Build history of the part. All positions in model axes, mm. A direction names the side the tool comes from. Round coordinates to 2 decimals unless told otherwise and drop trailing zeros. Write each loop counter-clockwise with the first axis right and the second up, starting at its lowest first coordinate (ties: lowest second). Pieces come first, ordered by that corner, then holes. Notation, with made-up numbers: (-35, -32.75) -> (-14, -32.75) arc R17 ccw to (-14, -1.75) -> close; hole circle Ø1 at (79, 69). An arc over 180 degrees is marked (long way). One line per question, with ' | ' between items.
from build123d import *

# Parameters (mm, degrees)
SKETCH1_R           = 11
SKETCH1_R_2         = 1.25
SKETCH1_R_3         = 2.5
SKETCH1_R_4         = 2.1
BOSS_EXTRUDE1_DEPTH = 2.5
FILLET1_R           = 0.5
FILLET2_R           = 2


with BuildPart() as part:
    # Sketch1 → Boss-Extrude1 (new, symmetric)
    with BuildSketch(Plane.XY):
        with BuildLine():
            Line((-30, -46), (-22.5, -46))
            Line((-22.5, -46), (-22.5, -45.3))
            ThreePointArc((-22.5, -45.3), (-23.8, -44), (-22.5, -42.7))
            Line((-22.5, -42.7), (-20.5, -42.7))
            ThreePointArc((-20.5, -42.7), (-19.2, -44), (-20.5, -45.3))
            Line((-20.5, -45.3), (-20.5, -46))
            Line((-20.5, -46), (20.5, -46))
            Line((20.5, -46), (20.5, -45.3))
            ThreePointArc((20.5, -45.3), (19.2, -44), (20.5, -42.7))
            Line((20.5, -42.7), (22.5, -42.7))
            ThreePointArc((22.5, -42.7), (23.8, -44), (22.5, -45.3))
            Line((22.5, -45.3), (22.5, -46))
            Line((22.5, -46), (30, -46))
            Line((30, -46), (30, 49))
            ThreePointArc((30, 49), (0, 79), (-30, 49))
            Line((-30, 49), (-30, -46))
        make_face()
        with Locations((0, -4.6)):
            Circle(SKETCH1_R, mode=Mode.SUBTRACT)
        with Locations((15.5, 10.9)):
            Circle(SKETCH1_R_2, mode=Mode.SUBTRACT)
        with Locations((15.5, -20.1)):
            Circle(SKETCH1_R_2, mode=Mode.SUBTRACT)
        with Locations((-15.5, -20.1)):
            Circle(SKETCH1_R_2, mode=Mode.SUBTRACT)
        with Locations((-15.5, 10.9)):
            Circle(SKETCH1_R_2, mode=Mode.SUBTRACT)
        with Locations((0, 49)):
            Circle(SKETCH1_R, mode=Mode.SUBTRACT)
        with Locations((21.5, -34)):
            Circle(SKETCH1_R_3, mode=Mode.SUBTRACT)
        with Locations((-21.5, -34)):
            Circle(SKETCH1_R_3, mode=Mode.SUBTRACT)
        with Locations((0, 64)):
            Circle(SKETCH1_R_4, mode=Mode.SUBTRACT)
        with Locations((-15, 49)):
            Circle(SKETCH1_R_4, mode=Mode.SUBTRACT)
        with Locations((0, 34)):
            Circle(SKETCH1_R_4, mode=Mode.SUBTRACT)
        with Locations((15, 49)):
            Circle(SKETCH1_R_4, mode=Mode.SUBTRACT)
        with Locations((20, 19.25)):
            Circle(SKETCH1_R_4, mode=Mode.SUBTRACT)
        with BuildLine():
            Line((20.5, -26.5), (22.5, -26.5))
            ThreePointArc((22.5, -26.5), (24, -28), (22.5, -29.5))
            Line((22.5, -29.5), (20.5, -29.5))
            ThreePointArc((20.5, -29.5), (19, -28), (20.5, -26.5))
        make_face(mode=Mode.SUBTRACT)
        with BuildLine():
            Line((-20.5, -26.5), (-22.5, -26.5))
            ThreePointArc((-22.5, -26.5), (-24, -28), (-22.5, -29.5))
            Line((-22.5, -29.5), (-20.5, -29.5))
            ThreePointArc((-20.5, -29.5), (-19, -28), (-20.5, -26.5))
        make_face(mode=Mode.SUBTRACT)
        with BuildLine():
            Line((-8.51843153, 12.888546871), (-18.855050358, 16.650768448))
            ThreePointArc((-18.855050358, 16.650768448), (-20.349231552, 19.855050358), (-17.144949642, 21.349231552))
            Line((-17.144949642, 21.349231552), (-6.808330813, 17.587009975))
            ThreePointArc((-6.808330813, 17.587009975), (-5.314149619, 14.382728065), (-8.51843153, 12.888546871))
        make_face(mode=Mode.SUBTRACT)
    extrude(amount=BOSS_EXTRUDE1_DEPTH, both=True)

    # Fillet1
    # the kernel refuses this fillet: 0.5 mm, written as the material it takes off along each edge
    with BuildSketch(Plane(origin=(-22.5, -46, -3.75), x_dir=(0, 1, 0), z_dir=(0, 0, 1)), Plane(origin=(-20.5, -46, -3.75), x_dir=(1, 0, 0), z_dir=(0, 0, 1)), Plane(origin=(20.5, -46, -3.75), x_dir=(0, 1, 0), z_dir=(0, 0, 1)), Plane(origin=(22.5, -46, -3.75), x_dir=(1, 0, 0), z_dir=(0, 0, 1))) as fillet1_piece_1:
        with BuildLine():
            CenterArc((FILLET1_R, FILLET1_R), FILLET1_R, 180, 90)
            Line((0, FILLET1_R), (0, 0))
            Line((0, 0), (FILLET1_R, 0))
        make_face()
    extrude(amount=7.5, mode=Mode.SUBTRACT)
    with BuildSketch(Plane(origin=(-22.5, -45.3, -3.572904116), x_dir=(-0.990112458059838, 0.14027587246103826, 0), z_dir=(0, 0, 1))) as fillet1_piece_2:
        with BuildLine():
            CenterArc((0.434855205, 0.495056229), FILLET1_R, 188.063810107, 73.872379787)
            Line((-0.060201024, 0.424918293), (0, 0))
            ThreePointArc((0, 0), (0.182358634, 0.012853805), (0.364717268, 0))
        make_face()
    extrude(amount=7.145808233, mode=Mode.SUBTRACT)
    with BuildSketch(Plane(origin=(-20.5, -45.3, -3.572904116), x_dir=(0, -1, 0), z_dir=(0, 0, 1))) as fillet1_piece_3:
        with BuildLine():
            CenterArc((0.429161647, 0.5), FILLET1_R, 196.127620213, 73.872379787)
            ThreePointArc((-0.051161033, 0.361111111), (-0.012853805, 0.182358634), (0, 0))
            Line((0, 0), (0.429161647, 0))
        make_face()
    extrude(amount=7.145808233, mode=Mode.SUBTRACT)
    with BuildSketch(Plane(origin=(20.5, -45.3, 3.572904116), x_dir=(-0.9901124580598404, 0.14027587246102047, 0), z_dir=(0, 0, -1)), Plane(origin=(22.5, -45.3, -3.572904116), x_dir=(0.9901124580598378, 0.1402758724610396, 0), z_dir=(0, 0, 1))) as fillet1_piece_4:
        with BuildLine():
            CenterArc((0.434855205, -0.495056229), FILLET1_R, 98.063810107, 73.872379787)
            Line((-0.060201024, -0.424918293), (0, 0))
            ThreePointArc((0, 0), (0.182358634, -0.012853805), (0.364717268, 0))
        make_face()
    extrude(amount=7.145808233, mode=Mode.SUBTRACT)

    # Fillet2
    fillet2_edges = [part.edges().sort_by_distance(p)[0] for p in [
        (30, -46, 0),
        (-30, -46, 0),
    ]]
    fillet(fillet2_edges, radius=FILLET2_R)


solid = part.part
(1) Wall check: line 1 (Y direction, x = 0, z = -0.7); line 2 (Y direction, x = 16, z = 0.3); line 3 (Y direction, x = -15.5, z = -0.85). Give the ranges that are in metal, low to high. Write a range as from..to.
Calculated:
line 1: -46..-15.6, 6.4..31.9, 36.1..38, 60..61.9, 66.1..79 | line 2: -46..-21.25, -18.95..9.75, 12.05..47.15, 50.85..74.38 | line 3: -46..-21.35, -18.85..9.65, 12.15..15.43, 20.75..46.96, 51.04..74.69
(2) Slice it at A-A (y = -28). Write the cut outline in (x, z).
Calculated:
outline: (-30, -2.5) -> (-24, -2.5) -> (-24, 2.5) -> (-30, 2.5) -> close; (-19, -2.5) -> (19, -2.5) -> (19, 2.5) -> (-19, 2.5) -> close; (24, -2.5) -> (30, -2.5) -> (30, 2.5) -> (24, 2.5) -> close
(3) Drop flat-ended pins along their axis: pin 1 (4.5 mm diameter, centred on x = -21.5, y = -34, fed in from +Z); pin 2 (3 mm diameter, centred on x = 15.5, y = 10.9, fed in from -Z); pin 3 (3 mm diameter, centred on y = 56, z = -0.5, fed in from +X); pin 4 (1 mm diameter, centred on x = -21, z = -1, fed in from +Y). Give the stop position or say it passes through.
Calculated:
pin 1: through | pin 2: z = -2.5 | pin 3: x = 29.49 | pin 4: y = 70.9
(4) Slice it at B-B (x = 0). Write the cut outline in (y, z).
Calculated:
outline: (-46, -2.5) -> (-15.6, -2.5) -> (-15.6, 2.5) -> (-46, 2.5) -> close; (6.4, -2.5) -> (31.9, -2.5) -> (31.9, 2.5) -> (6.4, 2.5) -> close; (36.1, -2.5) -> (38, -2.5) -> (38, 2.5) -> (36.1, 2.5) -> close; (60, -2.5) -> (61.9, -2.5) -> (61.9, 2.5) -> (60, 2.5) -> close; (66.1, -2.5) -> (79, -2.5) -> (79, 2.5) -> (66.1, 2.5) -> close
(5) Slice it at C-C (y = -0.5). Write the cut outline in (x, z), then the cut area to 3 significant figures.
Calculated:
outline: (-30, -2.5) -> (-10.21, -2.5) -> (-10.21, 2.5) -> (-30, 2.5) -> close; (10.21, -2.5) -> (30, -2.5) -> (30, 2.5) -> (10.21, 2.5) -> close | area: 198 mm2
(6) Slice it at D-D (x = 15.5). Write the cut outline in (y, z), then the cut area to 3 significant figures.
Calculated:
outline: (-46, -2.5) -> (-21.35, -2.5) -> (-21.35, 2.5) -> (-46, 2.5) -> close; (-18.85, -2.5) -> (9.65, -2.5) -> (9.65, 2.5) -> (-18.85, 2.5) -> close; (12.15, -2.5) -> (46.96, -2.5) -> (46.96, 2.5) -> (12.15, 2.5) -> close; (51.04, -2.5) -> (74.69, -2.5) -> (74.69, 2.5) -> (51.04, 2.5) -> close | area: 558 mm2
(7) 3-axis set-ups, long thin cutter, end or side, ignore diameter. For faces 1 (the flat face through (-13.61, 14.74, -0.04)), 2 (the flat face through (25, -46, 0)): which of +Z, -Z, +X, -X, +Y, -Y reach the whole face in a straight line?
Calculated:
face 1: +Z, -Z | face 2: +Z, -Z, +X, -X, -Y
(8) Mould opens along X. For faces 3 (the cylindrical face through (-8.11, 56.43, -0.04)), 4 (the flat face through (0, 17, -2.5)), 5 (the flat face through (30, 2, 0)) say: pulls with the +X half, pulls with the -X half, needs draft (parallel to the pull), parting line crosses it, or undercut.
Calculated:
face 3: undercut | face 4: needs draft | face 5: pulls with the +X half
